Design review of the part built by this model. Coordinates are the model's own, in mm. Face numbers are marked on the shaded views. A direction names the side the tool comes from. Coordinates: 2 decimals unless noted, no trailing zeros. Write each loop counter-clockwise with the first axis right and the second up, starting at its lowest first coordinate (ties: lowest second). Pieces come first, ordered by that corner, then holes. Notation, with made-up numbers: (89.5, -29) - (101.5, -29) arc R24 cw to (101.5, -19) - close; hole circle Ø9 at (5.5, 56.5). An arc over 180 degrees is marked (long way). Use a Markdown table: item, result.
from build123d import *

# Parameters (mm, degrees)
SKETCH1_W           = 44
SKETCH1_H           = 20
BOSS_EXTRUDE1_DEPTH = 2
SKETCH2_W           = 2.25
SKETCH2_H           = 20
BOSS_EXTRUDE2_DEPTH = 2
SKETCH3_W           = 4
SKETCH3_H           = 20
BOSS_EXTRUDE3_DEPTH = 1.5
SKETCH7_W           = 20
SKETCH7_H           = 2
BOSS_EXTRUDE4_DEPTH = 30
CHAMFER1_SIZE       = 30
CHAMFER1_SIZE2      = 17.320508076
SKETCH8_R           = 1.15
CUT_EXTRUDE1_DEPTH  = 39.522720569


with BuildPart() as part:
    # Sketch1 → Boss-Extrude1 (new body)
    with BuildSketch(Plane(origin=(0, 0, 0), x_dir=(1, 0, 0), z_dir=(0, 1, 0))):
        Rectangle(SKETCH1_W, SKETCH1_H)
    extrude(amount=BOSS_EXTRUDE1_DEPTH)

    # Sketch2 → Boss-Extrude2 (add)
    with BuildSketch(Plane(origin=(0, 2, 0), x_dir=(1, 0, 0), z_dir=(0, 1, 0))):
        with Locations((-20.875, 0)):
            Rectangle(SKETCH2_W, SKETCH2_H)
        with Locations((20.875, 0)):
            Rectangle(SKETCH2_W, SKETCH2_H)
    extrude(amount=BOSS_EXTRUDE2_DEPTH)

    # Sketch3 → Boss-Extrude3 (add)
    with BuildSketch(Plane(origin=(0, 4, 0), x_dir=(1, 0, 0), z_dir=(0, 1, 0))):
        with Locations((-20, 0)):
            Rectangle(SKETCH3_W, SKETCH3_H)
        with Locations((20, 0)):
            Rectangle(SKETCH3_W, SKETCH3_H)
    extrude(amount=BOSS_EXTRUDE3_DEPTH)

    # Sketch7 → Boss-Extrude4 (add)
    with BuildSketch(Plane.XZ):
        Polygon((-12, -10), (-10, -10), (-10, -8), (-10, 10), (-12, 10), align=None)
        with Locations((0, -9)):
            Rectangle(SKETCH7_W, SKETCH7_H)
        Polygon((10, -8), (10, -10), (11.784691828, -10), (11.784691828, 10), (10, 10), align=None)
    extrude(amount=BOSS_EXTRUDE4_DEPTH)

    # Chamfer1
    chamfer1_edges = [part.edges().sort_by_distance(p)[0] for p in [
        (10.892345914, -30, 10),
        (-11, -30, 10),
    ]]
    chamfer1_side = [part.faces().sort_by_distance(p)[0] for p in [
        (-21.434646129, 2.75, 10),
    ]]
    chamfer(chamfer1_edges, length=CHAMFER1_SIZE, length2=CHAMFER1_SIZE2, reference=chamfer1_side[0])

    # Sketch8 → Cut-Extrude1 (cut, through all)
    with BuildSketch(Plane.XZ):
        with Locations(Location((-0.107654086, -1.3, 0), (0, 0, 270))):
            Circle(SKETCH8_R)
    extrude(amount=-CUT_EXTRUDE1_DEPTH, mode=Mode.SUBTRACT)


solid = part.part
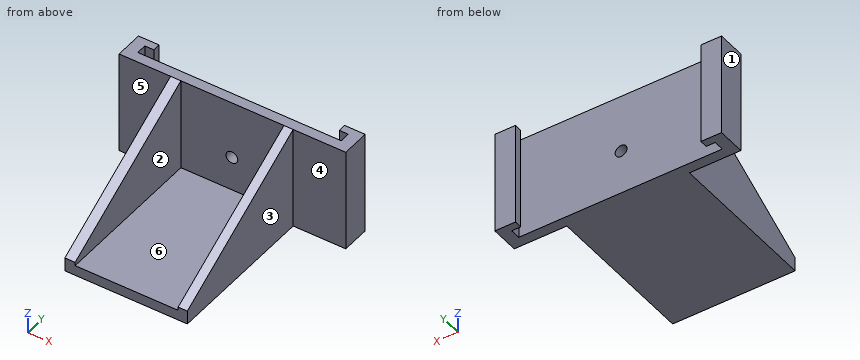
(1) For pin 1 (2.5 mm diameter, centred on x = -0.11, z = -1.3, fed in from +Y); pin 2 (3 mm diameter, centred on x = -18, z = -0.5, fed in from -Y); pin 3 (5 mm diameter, centred on x = -2, y = -24.5, fed in from +Z), all flat-tipped, find the tip position at first contact; note any pin that passes through.
Determined:
| item | result |
|---|---|
| pin 1 | y = 2 |
| pin 2 | y = 0 |
| pin 3 | z = -8 |
(2) Take a section at A-A on z = -0.75. Write out the cut boundary in (x, y), and give its area (3 significant figures).
Determined:
| item | result |
|---|---|
| outline | (-22, 0) - (-12, 0) - (-12, -18.62) - (-10, -18.62) - (-10, 0) - (-1.12, 0) - (-1.12, 2) - (-19.75, 2) - (-19.75, 4) - (-18, 4) - (-18, 5.5) - (-22, 5.5) - close; (0.9, 0) - (10, 0) - (10, -18.62) - (11.78, -18.62) - (11.78, 0) - (22, 0) - (22, 5.5) - (18, 5.5) - (18, 4) - (19.75, 4) - (19.75, 2) - (0.9, 2) - close |
| area | 175 mm2 |
(3) Draft analysis for pull direction X (two halves, no side actions). For the marked faces 1, 2 and 3, state which applies: +X half, -X half, draft (parallel to the pull), parting line (faces both ways), or undercut.
Determined:
| item | result |
|---|---|
| face 1 | -X half |
| face 2 | undercut |
| face 3 | +X half |
(4) Take a section at B-B on x = 6. Write out the cut boundary in (y, z).
Determined:
| item | result |
|---|---|
| outline | (-30, -10) - (2, -10) - (2, 10) - (0, 10) - (0, -8) - (-30, -8) - close |
(5) For L1, parallel to X at y = 0.55, z = -1.3; L2, parallel to Y at x = -18.5, z = 4; L3, parallel to X at y = -3, z = -6.5, list the stretches that pass through material, from the lowest coordinate up. Write a range as from..to.
Determined:
| item | result |
|---|---|
| L1 | -22..-1.26, 1.04..22 |
| L2 | 0..2, 4..5.5 |
| L3 | -12..-10, 10..11.78 |
(6) Machinability: for the marked faces 4, 5 and 6, which of the approach directions +Z, -Z, +X, -X, +Y, -Y give a long, thin tool a straight path to every point of the face, cutting with its end or side? Answer none if there is none.
Determined:
| item | result |
|---|---|
| face 4 | +Z, -Z, +X, -Y |
| face 5 | +Z, -Z, -X, -Y |
| face 6 | +Z, -Y |
(7) Take a section at C-C on z = 2.75. Write out the cut boundary in (x, y), and give its area (3 significant figures).
Determined:
| item | result |
|---|---|
| outline | (-22, 0) - (-12, 0) - (-12, -12.56) - (-10, -12.56) - (-10, 0) - (10, 0) - (10, -12.56) - (11.78, -12.56) - (11.78, 0) - (22, 0) - (22, 5.5) - (18, 5.5) - (18, 4) - (19.75, 4) - (19.75, 2) - (-19.75, 2) - (-19.75, 4) - (-18, 4) - (-18, 5.5) - (-22, 5.5) - close |
| area | 157 mm2 |
(8) Take a section at D-D on y = -26. Write out the cut boundary in (x, z).
Determined:
| item | result |
|---|---|
| outline | (-12, -10) - (11.78, -10) - (11.78, -5.01) - (10, -5.01) - (10, -8) - (-10, -8) - (-10, -5.01) - (-12, -5.01) - close |
